from build123d import *

# Parameters (mm, degrees)
BOSS_EXTRUDE1_DEPTH      = 25
BOSS_EXTRUDE1_DEPTH_BACK = 1
FILLET1_R                = 12.5
CUT_EXTRUDE3_DEPTH       = 132.655011329
CUT_EXTRUDE3_DEPTH_BACK  = 132.655011329
SKETCH3_R                = 7.5
FILLET4_R                = 2


with BuildPart() as part:
    # Sketch1 → Boss-Extrude1 (new, two sides: drawn at the far end of the back side and taken through both)
    with BuildSketch(Plane.YZ.offset(-BOSS_EXTRUDE1_DEPTH_BACK)):
        Polygon((-54.26996378, -10), (-54.26996378, 10), (-40.299013823, 10), (95.73003622, 30), (125.73003622, 30), (125.73003622, 15), (95.73003622, 15), (95.73003622, -15), (125.73003622, -15), (125.73003622, -30), (95.73003622, -30), (-40.299013823, -10), align=None)
        Polygon((25.73003622, -7.247706801), (25.73003622, 7.247706801), (75.73003622, 14.599077701), (75.73003622, -14.599077701), align=None, mode=Mode.SUBTRACT)
    extrude(amount=BOSS_EXTRUDE1_DEPTH + BOSS_EXTRUDE1_DEPTH_BACK)

    # Fillet1
    fillet1_edges = [part.edges().sort_by_distance(p)[0] for p in [
        (25, 125.73003622, -22.5),
        (25, -54.26996378, 0),
        (-1, 125.73003622, -22.5),
        (-1, -54.26996378, 0),
        (25, 125.73003622, 22.5),
        (-1, 125.73003622, 22.5),
    ]]
    fillet(fillet1_edges, radius=FILLET1_R)

    # Sketch3 → Cut-Extrude3 (cut, two sides: drawn at the far end of the back side and taken through both)
    with BuildSketch(Plane(origin=(0, 0, 0), x_dir=(0, 1, 0), z_dir=(0, 0, 1)).offset(-CUT_EXTRUDE3_DEPTH_BACK)):
        with Locations(Location((-40.299013823, -12, 0), (0, 0, 270))):
            Circle(SKETCH3_R)
        with Locations(Location((110.619547971, -12, 0), (0, 0, 270))):
            Circle(SKETCH3_R)
    extrude(amount=CUT_EXTRUDE3_DEPTH + CUT_EXTRUDE3_DEPTH_BACK, mode=Mode.SUBTRACT)

    # Fillet4
    fillet4_edges = [part.edges().sort_by_distance(p)[0] for p in [
        (12, 125.73003622, 15),
        (21.338834765, 122.068870985, 15),
        (2.661165235, 122.068870985, 15),
        (12, 125.73003622, 30),
        (21.338834765, 122.068870985, 30),
        (2.661165235, 122.068870985, 30),
        (25, 104.48003622, -30),
        (25, 27.715511199, -20),
        (25, 75.73003622, 0),
        (25, 50.73003622, 10.923392251),
        (25, 25.73003622, 0),
        (25, 50.73003622, -10.923392251),
        (25, 27.715511199, 20),
        (-1, 104.48003622, -30),
        (-1, 27.715511199, -20),
        (25, 104.48003622, 30),
        (-1, 50.73003622, -10.923392251),
        (-1, 95.73003622, 0),
        (-1, 27.715511199, 20),
        (-1, 104.48003622, 30),
        (-1, 25.73003622, 0),
        (-1, 50.73003622, 10.923392251),
        (-1, 75.73003622, 0),
        (-1, 104.48003622, 15),
        (-1, 104.48003622, -15),
        (-1, -41.034488801, -10),
        (-1, -41.034488801, 10),
        (12, -54.26996378, 10),
        (25, -41.034488801, 10),
        (21.338834765, -50.608798545, 10),
        (2.661165235, -50.608798545, 10),
        (12, -54.26996378, -10),
        (25, 95.73003622, 0),
        (25, -41.034488801, -10),
        (21.338834765, -50.608798545, -10),
        (2.661165235, -50.608798545, -10),
        (25, 104.48003622, 15),
        (25, 104.48003622, -15),
        (12, 125.73003622, -30),
        (12, 125.73003622, -15),
        (21.338834765, 122.068870985, -15),
        (2.661165235, 122.068870985, -15),
        (21.338834765, 122.068870985, -30),
        (2.661165235, 122.068870985, -30),
    ]]
    fillet(fillet4_edges, radius=FILLET4_R)


solid = part.part
Input: part model. Units: mm. Frame: model coordinates. A direction names the side the tool comes from. Give positions to 0.01 mm unless a question says otherwise; leave off trailing zeros. Write each loop counter-clockwise with the first axis right and the second up, starting at its lowest first coordinate (ties: lowest second). Pieces come first, ordered by that corner, then holes.
Q1. Material intervals for probe 1 along Y at (x, z) = (12, 2.5); probe 2 along Y at (x, z) = (16.25, 1); probe 3 along Z at (x, y) = (7.5, 104), sorted ascending.
Q2. Pull-direction query (Z, two-part tool) for faces 1 (the face through (7, 104, 15)), 2 (the face through (11.024, -32.863, -0.169)), 3 (the face through (11.85, 26.76, 19.86)); classes: pulls with the +Z half, pulls with the -Z half, needs draft (parallel to the pull), parting line crosses it, or undercut.
Q3. First-contact query: P1, Ø1.5, axis at x = 21, y = 12.5, coming from the +Z side; P2, Ø8, axis at x = 4, z = 4, coming from the -Y side; P3, Ø6, axis at x = 5.5, y = 70.5, coming from the +Z side; P4, Ø6.5, axis at x = 11, y = 105, coming from the -Z side. Flat tips, straight axial feed; report the tip coordinate or a pass-through.
Q4. Set-up query: faces 4 (the face through (12, -49, -10)), 5 (the face through (9, 103, -15)), 6 (the face through (12, 75.73, 0)), 7 (the face through (-0.43, 50.555, -11.506)). Return all of +Z, -Z, +X, -X, +Y, -Y with unobstructed straight access to the full face (end or side cutting, diameter ignored); none if empty.
Q5. Section B-B, the plane x = 17.5. State how many separate pieces and enclosed holes the cut face has, plus the area to 3 significant figures.
Q6. Section A-A, the plane z = -3.5. Output: boundary loops of the cut face in (x, y).
Filled in:
1. probe 1: y = -54.27 to -47.8, -32.8 to 25.73, 75.73 to 95.73
1. probe 2: y = -53.69 to -46.48, -34.12 to 25.73, 75.73 to 95.73
1. probe 3: z = -30 to -15, 15 to 30
2. face 1: undercut
2. face 2: needs draft
2. face 3: pulls with the +Z half
3. P1: stops at z = 17.87
3. P2: stops at y = -53.77
3. P3: stops at z = 26.73
3. P4: stops at z = -30
4. face 4: -Z, +X, -X, -Y
4. face 5: +X, -X, +Y
4. face 6: +X, -X
4. face 7: -X
5. separate pieces: 4
5. enclosed holes: 1
5. area: 4,960 mm2
6. outline: (-1, -41.77) arc R12.5 ccw to (11.5, -54.27) - (12.5, -54.27) arc R12.5 ccw to (25, -41.77) - (25, 23.73) arc R2 ccw to (23, 25.73) - (1, 25.73) arc R2 ccw to (-1, 23.73) - close; (-1, 77.73) arc R2 ccw to (1, 75.73) - (23, 75.73) arc R2 ccw to (25, 77.73) - (25, 93.73) arc R2 ccw to (23, 95.73) - (1, 95.73) arc R2 ccw to (-1, 93.73) - close; hole circle Ø15 at (12, -40.3)
